from build123d import *

# Parameters (mm, degrees)
SKETCH1_R           = 14
SKETCH1_R_2         = 1.65
BOSS_EXTRUDE1_DEPTH = 14
SKETCH2_R           = 14
SKETCH2_R_2         = 4
CUT_EXTRUDE1_DEPTH  = 9.5
SKETCH3_R           = 14
SKETCH3_R_2         = 7.5
CUT_EXTRUDE2_DEPTH  = 1
CUT_EXTRUDE3_DEPTH  = 4.5


with BuildPart() as part:
    # Sketch1 → Boss-Extrude1 (new body)
    with BuildSketch(Plane.XY):
        Circle(SKETCH1_R)
        Circle(SKETCH1_R_2, mode=Mode.SUBTRACT)
    extrude(amount=BOSS_EXTRUDE1_DEPTH)

    # Sketch2 → Cut-Extrude1 (cut)
    with BuildSketch(Plane.XY.offset(14)):
        Circle(SKETCH2_R)
        Circle(SKETCH2_R_2, mode=Mode.SUBTRACT)
    extrude(amount=-CUT_EXTRUDE1_DEPTH, mode=Mode.SUBTRACT)

    # Sketch3 → Cut-Extrude2 (cut)
    with BuildSketch(Plane.XY.offset(4.5)):
        Circle(SKETCH3_R)
        Circle(SKETCH3_R_2, mode=Mode.SUBTRACT)
    extrude(amount=-CUT_EXTRUDE2_DEPTH, mode=Mode.SUBTRACT)

    # Sketch4 → Cut-Extrude3 (cut, through all)
    with BuildSketch(Plane.XY.offset(3.5)):
        with BuildLine():
            Line((6.495190528, 3.75), (12.124355653, 7))
            ThreePointArc((12.124355653, 7), (0, 14), (-12.124355653, 7))
            Line((-12.124355653, 7), (-6.495190528, 3.75))
            ThreePointArc((-6.495190528, 3.75), (0, 7.5), (6.495190528, 3.75))
        make_face()
    extrude(amount=-CUT_EXTRUDE3_DEPTH, mode=Mode.SUBTRACT)


solid = part.part
Source: CAD feature listing. Evaluate the final solid. Frame: model axes, mm. A direction names the side the tool comes from. Round coordinates to 2 decimals unless told otherwise and drop trailing zeros. Loops run counter-clockwise (first coordinate to the right, second up) from the corner with the lowest first, then second, coordinate; pieces in that order, holes last.
Q1. Mould query, pull axis Y, two halves, no side actions, for faces 1 (the face through (2, 0, 14)), 2 (the face through (-0.867, -3.905, 9.317)), 3 (the face through (-1.216, 1.115, 6.902)). Classes: pulls with the +Y half, pulls with the -Y half, needs draft (parallel to the pull), parting line crosses it, or undercut.
Q2. Section D-D, the plane y = 2.75. Return loops of the section in (x, z).
Q3. Ray query, line 1 (Y direction, x = 0, z = 10.75); line 2 (Z direction, x = -2, y = -8.5); line 3 (Y direction, x = 0, z = 4). Return the intervals inside material, ascending.
Q4. Section B-B, the plane x = 0. Return loops of the section in (y, z), plus the area to 3 significant figures.
Q5. Section A-A, the plane y = 0. Return loops of the section in (x, z), plus the area to 3 significant figures.
Q6. First-contact query: P1, Ø1, axis at x = 10, y = -9, coming from the +Z side; P2, Ø6, axis at x = 5, z = 12.5, coming from the -Y side; P3, Ø12, axis at x = 8.5, y = -0.5, coming from the -Z side. Flat tips, straight axial feed; report the tip coordinate or a pass-through.
Q7. Access query for faces 4 (the face through (0, -14, 2)), 5 (the face through (3, -3, 4.5)), 6 (the face through (9.27, 5.35, 1.77)). Directions: +Z, -Z, +X, -X, +Y, -Y. A direction counts if a zero-diameter tool reaches every point of the face in a straight line with its end or side. Return the directions, or none.
Q8. Section C-C, the plane z = 13. Return loops of the section in (x, y).
Solutions:
1. face 1: needs draft
1. face 2: parting line crosses it
1. face 3: undercut
2. outline: (-13.73, 0) - (13.73, 0) - (13.73, 3.5) - (6.98, 3.5) - (6.98, 4.5) - (2.9, 4.5) - (2.9, 14) - (-2.9, 14) - (-2.9, 4.5) - (-6.98, 4.5) - (-6.98, 3.5) - (-13.73, 3.5) - close
3. line 1: y = -4 to -1.65, 1.65 to 4
3. line 2: z = 0 to 3.5
3. line 3: y = -7.5 to -1.65, 1.65 to 7.5
4. outline: (-14, 0) - (-1.65, 0) - (-1.65, 14) - (-4, 14) - (-4, 4.5) - (-7.5, 4.5) - (-7.5, 3.5) - (-14, 3.5) - close; (1.65, 0) - (7.5, 0) - (7.5, 4.5) - (4, 4.5) - (4, 14) - (1.65, 14) - close
4. area: 120 mm2
5. outline: (-14, 0) - (-1.65, 0) - (-1.65, 14) - (-4, 14) - (-4, 4.5) - (-7.5, 4.5) - (-7.5, 3.5) - (-14, 3.5) - close; (1.65, 0) - (14, 0) - (14, 3.5) - (7.5, 3.5) - (7.5, 4.5) - (4, 4.5) - (4, 14) - (1.65, 14) - close
5. area: 143 mm2
6. P1: stops at z = 3.5
6. P2: stops at y = -3.46
6. P3: stops at z = 0
7. face 4: +Z, -Z
7. face 5: +Z
7. face 6: +Z, -Z, +Y
8. outline: circle Ø8 at (0, 0); hole circle Ø3.3 at (0, 0)
